Work out the finished part from the listing and answer in its coordinate system (mm). A direction names the side the tool comes from. Coordinates: 2 decimals unless noted, no trailing zeros. Order: outer loops, then holes, each group sorted by start corner. A loop starts at its lowest first (then second) coordinate and runs counter-clockwise, first axis right, second up. Notation, with made-up numbers: M 59.25,22 L 86.25,22 A10 ccw 86.25,26 Z; hole C 71,32.25 d1. An arc over 180 degrees is marked long. Use a Markdown table: item, result.
from build123d import *

# Parameters (mm, degrees)
SKETCH2_R               = 61.9125
BOSS_EXTRUDE1_DEPTH     = 5
SKETCH3_R               = 32.5
SKETCH3_R_2             = 23.5
BOSS_EXTRUDE2_DEPTH     = 7
SKETCH6_R               = 14.85
BOSS_EXTRUDE3_DEPTH     = 2
CUT_EXTRUDE1_DEPTH      = 2
CUT_EXTRUDE1_DEPTH_BACK = 5
SKETCH5_R               = 1.25


with BuildPart() as part:
    # Sketch2 → Boss-Extrude1 (new body)
    with BuildSketch(Plane(origin=(0, 0, 0), x_dir=(1, 0, 0), z_dir=(0, 1, 0))):
        with Locations(Location((0, 0, 0), (0, 0, 270))):
            Circle(SKETCH2_R)
    extrude(amount=BOSS_EXTRUDE1_DEPTH)

    # Sketch3 → Boss-Extrude2 (add)
    with BuildSketch(Plane(origin=(0, 0, 0), x_dir=(1, 0, 0), z_dir=(0, 1, 0))):
        with Locations(Location((0, 0, 0), (0, 0, 270))):
            Circle(SKETCH3_R)
        with Locations(Location((0, 0, 0), (0, 0, 270))):
            Circle(SKETCH3_R_2, mode=Mode.SUBTRACT)
    extrude(amount=-BOSS_EXTRUDE2_DEPTH)

    # Sketch6 → Boss-Extrude3 (add)
    with BuildSketch(Plane(origin=(0, 0, 0), x_dir=(1, 0, 0), z_dir=(0, 1, 0))):
        with Locations(Location((0, 0, 0), (0, 0, 270))):
            Circle(SKETCH6_R)
    extrude(amount=-BOSS_EXTRUDE3_DEPTH)

    # Sketch5 → Cut-Extrude1 (cut, two sides: drawn at the far end of the back side and taken through both)
    with BuildSketch(Plane(origin=(0, 0, 0), x_dir=(-1, 0, 0), z_dir=(0, -1, 0)).offset(-CUT_EXTRUDE1_DEPTH_BACK)):
        with Locations(Location((0, 0, 0), (0, 0, 90))):
            Circle(SKETCH5_R)
        with Locations(Location((-4.058493048, -6.043759937, 0), (0, 0, 90))):
            Circle(SKETCH5_R)
        with Locations(Location((-6.043759937, 4.058493048, 0), (0, 0, 90))):
            Circle(SKETCH5_R)
        with Locations(Location((4.058493048, 6.043759937, 0), (0, 0, 90))):
            Circle(SKETCH5_R)
        with Locations(Location((6.043759937, -4.058493048, 0), (0, 0, 90))):
            Circle(SKETCH5_R)
    extrude(amount=CUT_EXTRUDE1_DEPTH + CUT_EXTRUDE1_DEPTH_BACK, mode=Mode.SUBTRACT)


solid = part.part
(1) Given P1, Ø1.5, axis at x = 4.06, z = 6.04, coming from the +Y side; P2, Ø1.5, axis at y = -2.5, z = -1.5, coming from the -X side; P3, Ø4, axis at y = 2.5, z = 6.5, coming from the -X side; P4, Ø6, axis at y = -1.5, z = -29, coming from the +X side, each flat-ended and moving along its own axis, determine where each tip first touches the part or whether it passes through.
Conclusion:
| item | result |
|---|---|
| P1 | through |
| P2 | x = -32.49 |
| P3 | x = -61.75 |
| P4 | x = 56 |
(2) A cutting plane is placed at C-C (x = -43.5). Determine the outline of the cut face in (y, z).
Conclusion:
| item | result |
|---|---|
| outline | M 0,-44.06 L 5,-44.06 L 5,44.06 L 0,44.06 Z |
(3) A cutting plane is placed at A-A (y = -3.75). Determine the outline of the cut face in (x, z), then the cut area to 3 significant figures.
Conclusion:
| item | result |
|---|---|
| outline | C 0,0 d65; hole C 0,0 d47 |
| area | 1,580 mm2 |
(4) Which of the six approach directions +Z, -Z, +X, -X, +Y, -Y give full straight-line access (tool end or side, diameter ignored) to faces 1 (the flat face through (-22, -7, 9)), 2 (the cylindrical face through (9.76, -3.45, 31))?
Conclusion:
| item | result |
|---|---|
| face 1 | +Z, -Z, +X, -X, -Y |
| face 2 | -Y |
(5) Straight lines are drawn through the part: L1, parallel to X at y = -2.25, z = 0; L2, parallel to Y at x = 44, z = -23; L3, parallel to X at y = 1.5, z = -0.5. For each, find the intervals that lie inside material, in ascending order.
Conclusion:
| item | result |
|---|---|
| L1 | -32.5 to -23.5, 23.5 to 32.5 |
| L2 | 0 to 5 |
| L3 | -61.91 to -1.15, 1.15 to 61.91 |
(6) A cutting plane is placed at D-D (z = -9.5). Determine the outline of the cut face in (x, y), then the cut area to 3 significant figures.
Conclusion:
| item | result |
|---|---|
| outline | M -61.18,0 L -31.08,0 L -31.08,-7 L -21.49,-7 L -21.49,0 L -11.41,0 L -11.41,-2 L 11.41,-2 L 11.41,0 L 21.49,0 L 21.49,-7 L 31.08,-7 L 31.08,0 L 61.18,0 L 61.18,5 L -61.18,5 Z |
| area | 792 mm2 |
(7) A cutting plane is placed at B-B (z = 27). Determine the outline of the cut face in (x, y), then the cut area to 3 significant figures.
Conclusion:
| item | result |
|---|---|
| outline | M -55.71,0 L -18.09,0 L -18.09,-7 L 18.09,-7 L 18.09,0 L 55.71,0 L 55.71,5 L -55.71,5 Z |
| area | 810 mm2 |
(8) Determine the mould class of faces 3 (the cylindrical face through (15.88, -3.45, -17.32)), 4 (the flat face through (-27, 0, 27)), 5 (the cylindrical face through (-60.44, 2.46, -13.42)), 6 (the flat face through (-3, -2, 0)) for opening direction X: pulls with the +X half, pulls with the -X half, needs draft (parallel to the pull), parting line crosses it, or undercut.
Conclusion:
| item | result |
|---|---|
| face 3 | undercut |
| face 4 | needs draft |
| face 5 | parting line crosses it |
| face 6 | undercut |
